Autodesk Inventor part; units mm, degrees
ref_plane "Work Plane1" through (0, -35.5, 0) normal (0, 1, 0) x (1, 0, 0)
ref_plane "Work Plane2" through (-9.7, -35.5, -10) normal (-1, 0, 0) x (0, 0, 1)
ref_plane "Work Plane3" through (-19.4, -35.5, 0) normal (0, 0, 1) x (1, 0, 0)
sketch "Sketch1" plane through (0, 0, 0) normal (0, 0, 1) x (1, 0, 0)
  arc A0 (68.484, -50.5) -> (70.5979, -47.5) centre (0, 0) ccw
  line L0 (0, -47.5) -> (70.5979, -47.5)
  line L1 (0, -47.5) -> (0, -50.5)
  line L2 (0, -50.5) -> (68.484, -50.5)
  dimension "d0" = 170.18
  dimension "d1" = 37.59
  dimension "d13" = 3
revolve "Revolution1" add sketch "Sketch1" angle 360 about axis through (0, -47.5, 0) along (0, -1, 0)
ref_plane "Work Plane1" through (0, -35.5, 0) normal (0, 1, 0) x (1, 0, 0)
sketch "Sketch2" plane through (0, -35.5, 0) normal (0, 1, 0) x (1, 0, 0)
  line L0 (10.3, -10) -> (-29.7, -10) construction
  line L1 (-29.7, -10) -> (-29.7, 10) construction
  line L2 (-29.7, 10) -> (10.3, 10) construction
  line L3 (10.3, 10) -> (10.3, -10) construction
  line L4 (0, 0) -> (-20, 0) construction
  line L5 (10.3, 10) -> (10.3, 7)
  line L6 (10.3, 7) -> (13.3, 7)
  line L7 (13.3, 7) -> (13.3, 13)
  line L8 (13.3, 13) -> (4.3, 13)
  line L9 (4.3, 13) -> (4.3, 10)
  line L10 (10.3, 10) -> (4.3, 10)
  line L11 (-9.7, 10) -> (-9.7, -10) construction
  line L12 (-19.4, 0) -> (0.6, 0) construction
  line L13 (-29.7, 10) -> (-29.7, 7)
  line L14 (-29.7, 7) -> (-32.7, 7)
  line L15 (-32.7, 7) -> (-32.7, 13)
  line L16 (-32.7, 13) -> (-23.7, 13)
  line L17 (-23.7, 13) -> (-23.7, 10)
  line L18 (-29.7, 10) -> (-23.7, 10)
  line L19 (10.3, -10) -> (10.3, -7)
  line L20 (10.3, -7) -> (13.3, -7)
  line L21 (13.3, -7) -> (13.3, -13)
  line L22 (13.3, -13) -> (4.3, -13)
  line L23 (4.3, -13) -> (4.3, -10)
  line L24 (10.3, -10) -> (4.3, -10)
  line L25 (-29.7, -10) -> (-29.7, -7)
  line L26 (-23.7, -13) -> (-23.7, -10)
  line L27 (-32.7, -13) -> (-23.7, -13)
  line L28 (-29.7, -7) -> (-32.7, -7)
  line L29 (-32.7, -7) -> (-32.7, -13)
  line L30 (-29.7, -10) -> (-23.7, -10)
  dimension "d3" = 40
  dimension "d4" = 20
  dimension "d5" = 20
  dimension "d6" = 29.7
  dimension "d7" = 3
  dimension "d8" = 3
  dimension "d9" = 6
  dimension "d10" = 9
sketch "Sketch4" plane through (0, 0, 0) normal (0, 0, 1) x (1, 0, 0)
  arc A0 (0, -85.09) -> (85.09, 0) centre (0, 0) ccw
  line L0 (0, -85.09) -> (0, 0) construction
  line L1 (0, 0) -> (85.09, 0) construction
  dimension "d28" = 170.18
surface revolve "RevolutionSrf1" sketch "Sketch4" angle 360 about axis through (0, -85.09, 0) along (0, 1, 0) shown yes curves A0
sketch "Sketch5" plane through (0, -47.5, 0) normal (0, 1, 0) x (1, 0, 0)
  circle A0 centre (-50, 0) radius 5
  circle A1 centre (-35.3553, -35.3553) radius 5
  circle A2 centre (0, -50) radius 5
  circle A3 centre (35.3553, -35.3553) radius 5
  circle A4 centre (50, 0) radius 5
  circle A5 centre (35.3553, 35.3553) radius 5
  circle A6 centre (0, 50) radius 5
  circle A7 centre (-35.3553, 35.3553) radius 5
  point P0 (0, 0)
  dimension "d38" = 10
  dimension "d39" = 50
  dimension "d42" = 360
extrude "Extrusion3" cut sketch "Sketch5" against normal through all
sketch "Sketch6" plane through (0, -47.5, 0) normal (0, 1, 0) x (1, 0, 0)
  line L0 (-23.7, 10) -> (-29.7, 10)
  line L1 (-23.7, 10) -> (-23.7, 16)
  line L2 (-23.7, 16) -> (-35.7, 16)
  line L3 (-35.7, 16) -> (-35.7, 7)
  line L4 (-29.7, 7) -> (-29.7, 10)
  line L5 (-35.7, 7) -> (-29.7, 7)
  line L6 (-29.7, 7) -> (-29.7, 10)
  line L7 (-9.7, 10) -> (-9.7, -10) construction
  line L8 (-19.4, 0) -> (0.6, 0) construction
  point P0 (0, 0)
  dimension "d46" = 6
  dimension "d47" = 12
  dimension "d48" = 9
  dimension "d49" = 90
sketch "Sketch7" plane through (0, -35.5, 0) normal (0, 1, 0) x (1, 0, 0)
  line L0 (-29.7, 10) -> (-23.7, 10)
  line L1 (-23.7, 10) -> (-23.7, 13)
  line L2 (-23.7, 13) -> (-32.7, 13)
  line L3 (-32.7, 13) -> (-32.7, 7)
  line L4 (-32.7, 7) -> (-29.7, 7)
  line L5 (-29.7, 7) -> (-29.7, 10)
  point P0 (0, 0)
  dimension "d51" = 6
  dimension "d52" = 3
  dimension "d53" = 90
  dimension "d54" = 9
  dimension "d55" = 90
  dimension "d56" = 6
  dimension "d57" = 3
sketch "Sketch8" plane through (0, -35.5, 0) normal (0, 1, 0) x (1, 0, 0)
  point P0 (0, 0)
loft "Loft1" add profiles "Sketch6", "Sketch7"
ref_plane "Work Plane2" through (-9.7, -35.5, -10) normal (-1, 0, 0) x (0, 0, 1)
ref_plane "Work Plane3" through (-19.4, -35.5, 0) normal (0, 0, 1) x (1, 0, 0)
mirror "Mirror1" about plane through (-9.7, -35.5, -10) normal (-1, 0, 0) of "Loft1"
mirror "Mirror2" about plane through (-19.4, -35.5, 0) normal (0, 0, 1) of "Loft1", "Mirror1"
properties part number "bottom_platform"
Model file for the job. Use its own axes, mm. A direction names the side the tool comes from. Coordinates: 2 decimals unless noted, no trailing zeros. Return JSON: item names as keys, results as strings.
1. Saw through at A-A (z = 0). Give the number of separate pieces and of enclosed holes in the cut face, and give its area (3 significant figures).
Ans:
{"separate pieces": "3", "enclosed holes": "0", "area": "357 mm^2"}
2. Tool access for faces 1 (the face through (7, -41, -10)), 2 (the face through (39.974, -48.979, -33.44)): list every direction of +Z, -Z, +X, -X, +Y, -Y with a clear straight run to the whole face (end or side of a thin tool).
Ans:
{"face 1": "+Y", "face 2": "+Y, -Y"}
3. Flat gauge pins, fed straight in: pin 1 (1 mm diameter, centred on x = 19, z = -37.5, fed in from +Y); pin 2 (2.5 mm diameter, centred on y = -39.5, z = 9, fed in from +X); pin 3 (5 mm diameter, centred on x = 6, y = -42.5, fed in from +Z) (3 decimals). Where does each tip first touch, or does it go through?
Ans:
{"pin 1": "y = -47.5", "pin 2": "x = 14.61", "pin 3": "z = 15.375"}
4. Drill centre lines: probe 1 along Z at (x, y) = (0, -49.1); probe 2 along Y at (x, z) = (36.5, -48.5); probe 3 along X at (y, z) = (-48.75, 48.5). Where is each one in solid material? Low to high.
Ans:
{"probe 1": "-69.49 to -55, -45 to 45, 55 to 69.49", "probe 2": "-50.5 to -47.5", "probe 3": "-50.11 to -4.77, 4.77 to 50.11"}
5. Pull direction X, two halves, no side cores. Call faces 3 (the face through (-33.05, -48.98, -30.92)), 4 (the face through (-1, -50.5, 1)): +X half, -X half, draft (parallel to the pull), parting line (faces both ways), or undercut.
Ans:
{"face 3": "undercut", "face 4": "draft"}
